Design review of the part built by this model. Coordinates are the model's own, in mm. A direction names the side the tool comes from. Coordinates: 2 decimals unless noted, no trailing zeros. Order: outer loops, then holes, each group sorted by start corner. A loop starts at its lowest first (then second) coordinate and runs counter-clockwise, first axis right, second up. Notation, with made-up numbers: (20.5, 30) -> (62.5, 30) arc R34 ccw to (62.5, 67) -> close; hole circle Ø8 at (-37, 60). An arc over 180 degrees is marked (long way). Use a Markdown table: item, result. Add a question column.
Q1. The part is to be moulded in two halves that separate along Z. For faces 1 (the face through (-2.635, 6.028, 2.681)), 2 (the face through (-11.4, 9, -24.8)), 3 (the face through (-2, 9, -16)), 4 (the face through (-9, 3, -18)), say which applies: pulls with the +Z half, pulls with the -Z half, needs draft (parallel to the pull), parting line crosses it, or undercut.
Q2. Machinability: for faces 5 (the face through (-6, 4, 1)), 6 (the face through (-16, 9, -16)), 7 (the face through (-9.1, 7, -19.6)), which of the approach directions +Z, -Z, +X, -X, +Y, -Y give a long, thin tool a straight path to every point of the face, cutting with its end or side? Answer none if there is none.
Q3. Add section C-C (y = 9.25). State the section outline as (x, z) points, then the cut area to 3 significant figures.
Q4. Add section B-B (z = -13). State the section outline as (x, y) points, then the cut area to 3 significant figures.
Q5. Insertion check: pin 1 (2 mm diameter, centred on x = -14.5, y = 5.5, fed in from -Z); pin 2 (5 mm diameter, centred on x = -10.5, y = 9.5, fed in from -Z); pin 3 (5 mm diameter, centred on x = -14, z = -3.5, fed in from +Y); pin 4 (1.8 mm diameter, centred on x = -8, z = -1, fed in from +Y). Each pin has a flat end and moves straight along its axis. Give the tip position at first contact, or say it passes through.
Q6. Add section D-D (x = -9). State the section outline as (y, z) points.
Q7. Wall thickness on probe 1 along Z at (x, y) = (-8.75, 5.5); probe 2 along Z at (x, y) = (-9, 9.15); probe 3 along X at (y, z) = (4.75, -13): over which ranges is each line inside the solid? List them lowest first.
Q8. Add section A-A (y = 6). State the section outline as (x, z) points.
Autodesk Inventor part; units mm, degrees
ref_plane "YZ Plane" through (0, 0, 0) normal (1, 0, 0) x (0, 1, 0)
ref_plane "XZ Plane" through (0, 0, 0) normal (0, 1, 0) x (-1, 0, 0)
ref_plane "XY Plane" through (0, 0, 0) normal (0, 0, 1) x (1, 0, 0)
sketch "Sketch1" plane through (0, 0, 0) normal (0, 1, 0) x (-1, 0, 0)
  line L0 (18, 0) -> (18, -30)
  line L1 (18, -30) -> (0, -30)
  line L2 (0, -30) -> (0, 0)
  arc A0 (18, 0) -> (0, 0) centre (9, 0) ccw
  circle A1 centre (9, -23) radius 1
  circle A2 centre (9, -13) radius 1
  dimension "d6" = 2
  dimension "d8" = 2
extrude "Extrusion1" add sketch "Sketch1" along normal blind 8
sketch "Sketch2" plane through (0, 8, 0) normal (0, 1, 0) x (1, 0, 0)
  circle A0 centre (-9.1017, 0) radius 3
  circle A1 centre (-9.1017, 0) radius 7
  point P0 (0, 0)
  dimension "d11" = 6
  dimension "d12" = 14
extrude "Extrusion2" cut sketch "Sketch2" against normal blind 4
sketch "Sketch3" plane through (-9.1017, 8, 0) normal (0, 1, 0) x (1, 0, 0)
  circle A0 centre (0, 0) radius 3
  point P0 (9.1017, 0)
extrude "Extrusion3" cut sketch "Sketch3" against normal blind 1.5
sketch "Sketch4" plane through (0, 8, 0) normal (0, 1, 0) x (1, 0, 0)
  line L0 (0, 23) -> (0, 16)
  line L1 (0, 16) -> (-18, 16)
  line L2 (-18, 16) -> (-18, 23)
  circle A0 centre (-9, 23) radius 3
  arc A1 (0, 23) -> (-18, 23) centre (-9, 17.5917) ccw
  point P0 (0, 0)
  dimension "d17" = 18
extrude "Extrusion4" add sketch "Sketch4" along normal blind 3
sketch "Sketch6" plane through (0, 0, 0) normal (0, -1, 0) x (1, 0, 0)
  line L0 (0, 0) -> (0, -30)
  line L1 (-18, -30) -> (-18, 0)
  line L2 (0, -30) -> (-18, -30)
  line L3 (-18, -30) -> (-18, -18)
  line L4 (-18, -18) -> (0, -18)
  line L5 (0, -18) -> (0, -30)
  dimension "d23" = 12
extrude "Extrusion5" cut sketch "Sketch6" against normal blind 7
sketch "Sketch7" plane through (0, 8, 0) normal (0, 1, 0) x (1, 0, 0)
  circle A0 centre (-9, 23) radius 3
  point P0 (0, 0)
  point P1 (-18, 23)
  point P2 (0, 30)
  point P3 (-6, 23)
  point P4 (-12, 23)
extrude "Extrusion6" cut sketch "Sketch7" against normal through all
sketch "Sketch8" plane through (0, 8, 0) normal (0, 1, 0) x (1, 0, 0)
  line L0 (-18, 30) -> (-18, 23)
  arc A0 (0, 23) -> (-18, 23) centre (-9, 17.5917) ccw
  line L1 (0, 30) -> (-18, 30)
  line L2 (3.2096, 23) -> (3.2096, 32.8991)
  line L3 (3.2096, 32.8991) -> (-22.1602, 32.8991)
  line L4 (-22.1602, 32.8991) -> (-22.1602, 23)
  line L5 (-22.1602, 23) -> (-18, 23)
  line L6 (0, 23) -> (3.2096, 23)
  point P0 (0, 0)
extrude "Extrusion7" cut sketch "Sketch8" against normal blind 7
sketch "Sketch11" plane through (0, 11, 0) normal (0, 1, 0) x (1, 0, 0)
  circle A0 centre (-9, 13) radius 1
  circle A1 centre (-9, 13) radius 6
  point P0 (0, 0)
  dimension "d38" = 12
extrude "Extrusion9" cut sketch "Sketch11" against normal blind 3
properties part number "top hand base with 2 gears"
Established:
| question | item | result |
|---|---|---|
| 1 | face 1 | undercut |
| 1 | face 2 | undercut |
| 1 | face 3 | pulls with the +Z half |
| 1 | face 4 | pulls with the -Z half |
| 2 | face 5 | +Y |
| 2 | face 6 | +Z, +X, -X, +Y |
| 2 | face 7 | -Z, +X, -X, -Y |
| 3 | outline | (-18, -23) arc R10.5 ccw to (0, -23) -> (0, -16) -> (-3.8, -16) arc R6 cw to (-14.2, -16) -> (-18, -16) -> close; hole circle Ø6 at (-9, -23) |
| 3 | area | 140 mm^2 |
| 4 | outline | (-18, 0) -> (-10, 0) -> (-10, 8) -> (-18, 8) -> close; (-8, 0) -> (0, 0) -> (0, 8) -> (-8, 8) -> close |
| 4 | area | 128 mm^2 |
| 5 | pin 1 | z = -18 |
| 5 | pin 2 | z = -28.09 |
| 5 | pin 3 | y = 8 |
| 5 | pin 4 | y = 6.5 |
| 6 | outline | (0, -18) -> (7, -18) -> (7, -20) -> (11, -20) -> (11, -19) -> (8, -19) -> (8, -14) -> (0, -14) -> close; (0, -12) -> (8, -12) -> (8, -7) -> (4, -7) -> (4, -3) -> (6.5, -3) -> (6.5, 3) -> (4, 3) -> (4, 7) -> (8, 7) -> (8, 9) -> (0, 9) -> close; (7, -28.09) -> (11, -28.09) -> (11, -26) -> (7, -26) -> close |
| 7 | probe 1 | -18 to -13.97, -12.03 to -6.99, -2.98 to 2.98, 6.99 to 9 |
| 7 | probe 2 | -28.09 to -26, -20 to -19 |
| 7 | probe 3 | -18 to -10, -8 to 0 |
| 8 | outline | (-18, -18) -> (0, -18) -> (0, 0) arc R9 ccw to (-18, 0) -> close; circle Ø6 at (-9.1, 0); hole circle Ø14 at (-9.1, 0); hole circle Ø2 at (-9, -13) |
